Source: CAD feature listing. Evaluate the final solid. Frame: model axes, mm. Face numbers are marked on the shaded views. A direction names the side the tool comes from. Round coordinates to 2 decimals unless told otherwise and drop trailing zeros. Loops run counter-clockwise (first coordinate to the right, second up) from the corner with the lowest first, then second, coordinate; pieces in that order, holes last. Notation, with made-up numbers: (71.25, 67) -> (122.25, 67) arc R25 ccw to (122.25, 90) -> close; hole circle Ø5 at (26, 72.25). An arc over 180 degrees is marked (long way). Put each result on its own line as item: value. Start each with the question number.
1. Cut plane D-D (x = 21.5). Return the cut outline in (y, z), then the cut area to 3 significant figures.
2. Set-up query: the marked faces 1, 2 and 3. Return all of +Z, -Z, +X, -X, +Y, -Y with unobstructed straight access to the full face (end or side cutting, diameter ignored); none if empty.
3. Cut plane B-B (x = 40). Return the cut outline in (y, z), then the cut area to 3 significant figures.
4. Contact query for flat-ended pins moving along their axis: pin 1 (2 mm diameter, centred on x = 39.5, y = 1.5, fed in from -Z); pin 2 (4 mm diameter, centred on y = 2.5, z = -9, fed in from -X); pin 3 (1 mm diameter, centred on y = 3, z = -3.5, fed in from -X); pin 4 (2.5 mm diameter, centred on x = 40, z = 0, fed in from -Y). Output: stop coordinate, or through.
5. Material intervals for L1, parallel to X at y = 4.55, z = 0; L2, parallel to Y at x = 16, z = -1; L3, parallel to X at y = 7.5, z = -0.5, sorted ascending.
6. Cut plane C-C (z = 6.5). Return the cut outline in (x, y), then the cut area to 3 significant figures.
7. Cut plane A-A (y = 7.25). Return the cut outline in (x, z).
```python
from build123d import *

# Parameters (mm, degrees)
EXTRUDE_1_DEPTH     = 4
SKETCH_2_R          = 4.5
SKETCH_2_R_2        = 3
EXTRUDE_2_DEPTH     = 2.5
EXTRUDE_3_DEPTH     = 25
SKETCH_4_W          = 7
SKETCH_4_H          = 5
CUT_EXTRUDE_1_DEPTH = 57.621550668
SKETCH_5_W          = 7
SKETCH_5_H          = 5
CUT_EXTRUDE_2_DEPTH = 52.780787943
SKETCH_6_R          = 3
SKETCH_6_R_2        = 1.5
EXTRUDE_4_DEPTH     = 1


with BuildPart() as part:
    # 草图1 → 凸台-拉伸1 (new body)
    with BuildSketch(Plane(origin=(0, 0, 0), x_dir=(1, 0, 0), z_dir=(0, 1, 0))):
        with BuildLine():
            ThreePointArc((12.5, 0), (8.838834765, 8.838834765), (0, 12.5))
            ThreePointArc((0, 12.5), (-8.838834765, 8.838834765), (-12.5, 0))
            Line((-12.5, 0), (-1.5, 0))
            ThreePointArc((-1.5, 0), (0, 1.5), (1.5, 0))
            Line((1.5, 0), (12.5, 0))
        make_face()
        with BuildLine():
            ThreePointArc((0, -12.5), (8.838834765, -8.838834765), (12.5, 0))
            Line((12.5, 0), (1.5, 0))
            ThreePointArc((1.5, 0), (0, -1.5), (-1.5, 0))
            Line((-1.5, 0), (-12.5, 0))
            ThreePointArc((-12.5, 0), (-8.838834765, -8.838834765), (0, -12.5))
        make_face()
        with BuildLine():
            Line((50, 12.5), (0, 12.5))
            ThreePointArc((0, 12.5), (8.838834765, 8.838834765), (12.5, 0))
            Line((12.5, 0), (38.5, 0))
            ThreePointArc((38.5, 0), (40, 1.5), (41.5, 0))
            Line((41.5, 0), (50, 0))
            Line((50, 0), (50, 12.5))
        make_face()
        with BuildLine():
            Line((38.5, 0), (12.5, 0))
            ThreePointArc((12.5, 0), (8.838834765, -8.838834765), (0, -12.5))
            Line((0, -12.5), (50, -12.5))
            Line((50, -12.5), (50, 0))
            Line((50, 0), (41.5, 0))
            ThreePointArc((41.5, 0), (40, -1.5), (38.5, 0))
        make_face()
    extrude(amount=EXTRUDE_1_DEPTH)

    # 草图2 → 凸台-拉伸2 (add)
    with BuildSketch(Plane(origin=(0, 4, 0), x_dir=(1, 0, 0), z_dir=(0, 1, 0))):
        with Locations(Location((0, 0, 0), (0, 0, 270))):
            Circle(SKETCH_2_R)
        with Locations(Location((0, 0, 0), (0, 0, 270))):
            Circle(SKETCH_2_R_2, mode=Mode.SUBTRACT)
    extrude(amount=EXTRUDE_2_DEPTH)

    # 草图3 → 凸台-拉伸3 (add)
    with BuildSketch(Plane.XY.offset(12.5)):
        Polygon((33, 9), (47, 9), (50, 4), (30, 4), align=None)
    extrude(amount=-EXTRUDE_3_DEPTH)

    # 草图4 → 切除-拉伸1 (cut, through all)
    with BuildSketch(Plane.XY.offset(12.5)):
        with Locations((40, 6.5)):
            Rectangle(SKETCH_4_W, SKETCH_4_H)
    extrude(amount=-CUT_EXTRUDE_1_DEPTH, mode=Mode.SUBTRACT)

    # 草图5 → 切除-拉伸2 (cut, through all)
    with BuildSketch(Plane(origin=(0, 4, 0), x_dir=(1, 0, 0), z_dir=(0, 1, 0))):
        with Locations((40, -10)):
            Rectangle(SKETCH_5_W, SKETCH_5_H)
        with Locations((40, 10)):
            Rectangle(SKETCH_5_W, SKETCH_5_H)
    extrude(amount=-CUT_EXTRUDE_2_DEPTH, mode=Mode.SUBTRACT)

    # 草图6 → 凸台-拉伸4 (add)
    with BuildSketch(Plane(origin=(0, 4, 0), x_dir=(1, 0, 0), z_dir=(0, 1, 0))):
        with Locations(Location((0, 0, 0), (0, 0, 270))):
            Circle(SKETCH_6_R)
        with Locations(Location((0, 0, 0), (0, 0, 270))):
            Circle(SKETCH_6_R_2, mode=Mode.SUBTRACT)
    extrude(amount=EXTRUDE_4_DEPTH)


solid = part.part
```
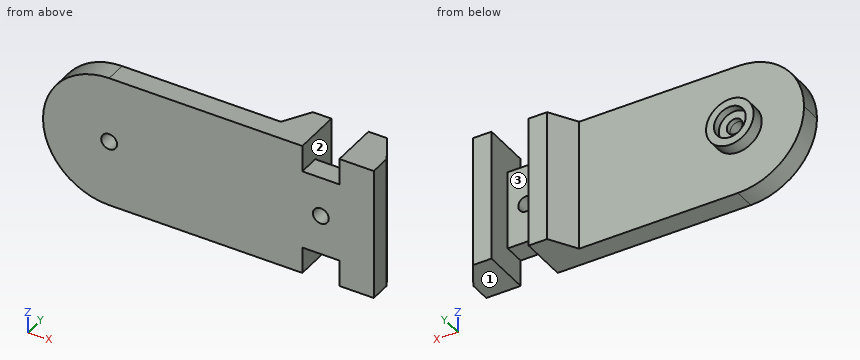
Solution:
1. outline: (0, -12.5) -> (4, -12.5) -> (4, 12.5) -> (0, 12.5) -> close
1. area: 100 mm^2
2. face 1: -Z, +X, -X, +Y, -Y
2. face 2: +Y
2. face 3: +Z, -Z, +Y
3. outline: (0, -7.5) -> (4, -7.5) -> (4, -1.5) -> (0, -1.5) -> close; (0, 1.5) -> (4, 1.5) -> (4, 7.5) -> (0, 7.5) -> close
3. area: 48.0 mm^2
4. pin 1: stops at z = -7.5
4. pin 2: stops at x = -10.36
4. pin 3: stops at x = -12.13
4. pin 4: passes through
5. L1: x = -4.5 to -1.5, 1.5 to 4.5, 30.33 to 36.5, 43.5 to 49.67
5. L2: y = 0 to 4
5. L3: x = 32.1 to 36.5, 43.5 to 47.9
6. outline: (-10.68, 0) -> (50, 0) -> (50, 4) -> (47, 9) -> (43.5, 9) -> (43.5, 4) -> (36.5, 4) -> (36.5, 9) -> (33, 9) -> (30, 4) -> (-10.68, 4) -> close
6. area: 293 mm^2
7. outline: (31.95, -12.5) -> (36.5, -12.5) -> (36.5, 12.5) -> (31.95, 12.5) -> close; (43.5, -12.5) -> (48.05, -12.5) -> (48.05, 12.5) -> (43.5, 12.5) -> close
